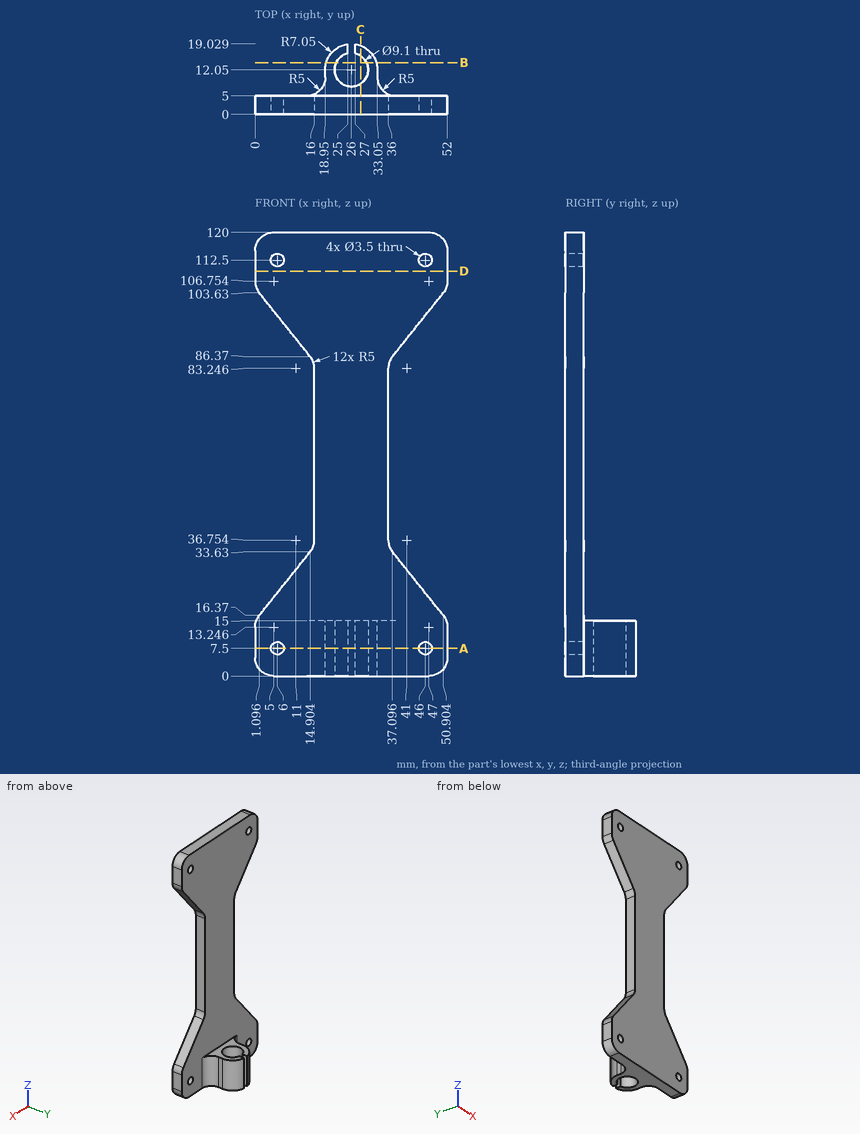
For this review, use the dimensioned drawing (mm, ordinates from the lowest corner) and the shaded views. Round coordinates to 2 decimals unless told otherwise and drop trailing zeros. Write each loop counter-clockwise with the first axis right and the second up, starting at its lowest first coordinate (ties: lowest second). Pieces come first, ordered by that corner, then holes. Notation, with made-up numbers: (23, -32) -> (43, -32) arc R19 cw to (43, -4) -> close; hole circle Ø4 at (39, 50.25). An arc over 180 degrees is marked (long way). Answer in a Markdown table with one row per item.
Q1. Take a section at A-A, the plane z = 7.5. State the section outline as (x, y) points.
The answers:
| item | result |
|---|---|
| outline | (0, 0) -> (4.25, 0) -> (4.25, 5) -> (0, 5) -> close; (7.75, 0) -> (44.25, 0) -> (44.25, 5) -> (38.05, 5) arc R5 cw to (33.05, 10) -> (33.05, 12.05) arc R7.05 ccw to (27, 19.03) -> (27, 16.49) arc R4.55 cw (long way) to (25, 16.49) -> (25, 19.03) arc R7.05 ccw to (18.95, 12.05) -> (18.95, 10) arc R5 cw to (13.95, 5) -> (7.75, 5) -> close; (47.75, 0) -> (52, 0) -> (52, 5) -> (47.75, 5) -> close |
Q2. Take a section at D-D, the plane z = 109.5. State the section outline as (x, y) points, then the cut area to 3 significant figures.
The answers:
| item | result |
|---|---|
| outline | (0, 0) -> (52, 0) -> (52, 5) -> (0, 5) -> close |
| area | 260 mm² |
Q3. Take a section at C-C, the plane x = 28.5. State the section outline as (y, z) points.
The answers:
| item | result |
|---|---|
| outline | (0, 0) -> (8.25, 0) -> (8.25, 15) -> (5, 15) -> (5, 120) -> (0, 120) -> close; (15.85, 0) -> (18.64, 0) -> (18.64, 15) -> (15.85, 15) -> close |
Q4. Take a section at B-B, the plane y = 14. State the section outline as (x, z) points (1 decimal).
The answers:
| item | result |
|---|---|
| outline | (19.2, 0) -> (21.9, 0) -> (21.9, 15) -> (19.2, 15) -> close; (30.1, 0) -> (32.8, 0) -> (32.8, 15) -> (30.1, 15) -> close |
Q5. To check wall thickness, follow L1, parallel to X at y = 3.45, z = 112.5; L2, parallel to Z at x = 46, y = 2.7; L3, parallel to X at y = 12.05, z = 7.25. State the ranges of each line that lie inside material, in increasing order. Write a range as [from, to].
The answers:
| item | result |
|---|---|
| L1 | [0, 4.25], [7.75, 44.25], [47.75, 52] |
| L2 | [0, 5.75], [9.25, 22.5], [97.5, 110.75], [114.25, 120] |
| L3 | [18.95, 21.45], [30.55, 33.05] |
Q6. Clearance check with flat-ended pins moving along their axes: pin 1 Ø3 at (x, z) = (6, 7.5) entering from -Y; pin 2 Ø5 at (x, y) = (34, 15.5) entering from +Z; pin 3 Ø6 at (y, z) = (7, 54.5) entering from -X; pin 4 Ø0.6 at (y, z) = (11.5, 4) entering from -X. State where each tip first meets the part, or that it passes through.
The answers:
| item | result |
|---|---|
| pin 1 | through |
| pin 2 | z = 15 |
| pin 3 | x = 16 |
| pin 4 | x = 18.95 |
